For this review, take the finished solid that the model builds, in its own axes (mm). A direction names the side the tool comes from. Coordinates: 2 decimals unless noted, no trailing zeros. Write each loop counter-clockwise with the first axis right and the second up, starting at its lowest first coordinate (ties: lowest second). Pieces come first, ordered by that corner, then holes. Notation, with made-up numbers: (33.25, 55.5) - (39.25, 55.5) arc R33 ccw to (39.25, 88.5) - close; hole circle Ø10 at (52.5, 40). An arc over 180 degrees is marked (long way). Use one line per item in the form item = value. Start each with the question number.
1) We need section C-C (x = 49.5). Give the boundary of the cut face in (y, z).
2) We need section B-B (z = -62). Give the boundary of the cut face in (x, y).
3) Mouldability with a two-part tool opening along X and no side actions: class faces 4 (the cylindrical face through (78.266, 1.521, 80.781)), 5 (the flat face through (1, 0, -1)), 6 (the cylindrical face through (-96.37, 1.48, 72.2)) as pulls with the +X half, pulls with the -X half, needs draft (parallel to the pull), parting line crosses it, or undercut.
4) For L1, parallel to X at y = 0.7, z = -56.5; L2, parallel to X at y = 2.1, z = 62; L3, parallel to X at y = 2.6, z = 23, list the stretches that pass through material, from the lowest coordinate up. Write a range as from..to.
5) We need section A-A (y = 1.35). Give the boundary of the cut face in (x, z).
6) Tool access review of faces 1 (the cylindrical face through (4.322, 1.521, 81.022)), 2 (the cylindrical face through (-4.314, 1.521, -81.101)), 3 (the flat face through (1, 3, -1)): name each direction out of +Z, -Z, +X, -X, +Y, -Y from which nothing blocks a thin tool from reaching the whole face with its end or side.
7) Insertion check: P1, Ø1.5, axis at x = -36.5, y = 2, coming from the -Z side; P2, Ø1.5, axis at y = 2, z = 13, coming from the +X side; P3, Ø1.5, axis at y = 1.5, z = -15, coming from the -X side. Each pin has a flat end and moves straight along its axis. Give the tip position at first contact, or say it passes through.
```python
from build123d import *

# Parameters (mm, degrees)
BOSS_EXTRUDE1_DEPTH = 3
FILLET1_R           = 5.08
FILLET2_R           = 5.08
FILLET3_R           = 5.08


with BuildPart() as part:
    # Sketch1 → Boss-Extrude1 (new body)
    with BuildSketch(Plane(origin=(0, 0, 0), x_dir=(1, 0, 0), z_dir=(0, 1, 0))):
        with BuildLine():
            Line((-76.2, 82.55), (-76.2, 55.95))
            Line((-76.2, 55.95), (-5.842, 55.95))
            Line((-5.842, 55.95), (-5.842, 82.55))
            Line((-5.842, 82.55), (5.770221656, 82.55))
            Line((5.770221656, 82.55), (5.770221656, 55.949868395))
            Line((5.770221656, 55.949868395), (76.2, 55.95))
            Line((76.2, 55.95), (76.2, 82.55))
            ThreePointArc((76.2, 82.55), (94.40904038, 74.510512242), (101.6, 55.95))
            Line((101.6, 55.95), (101.6, -55.95))
            ThreePointArc((101.6, -55.95), (94.40904038, -74.510512242), (76.2, -82.55))
            Line((76.2, -82.55), (76.2, -55.95))
            Line((76.2, -55.95), (5.770221656, -55.95))
            Line((5.770221656, -55.95), (5.770221656, -82.55))
            Line((5.770221656, -82.55), (-5.842, -82.55))
            Line((-5.842, -82.55), (-5.842, -55.95))
            Line((-5.842, -55.95), (-76.2, -55.95))
            Line((-76.2, -55.95), (-76.2, -82.55))
            ThreePointArc((-76.2, -82.55), (-94.40904038, -74.510512242), (-101.6, -55.95))
            Line((-101.6, -55.95), (-101.6, 55.95))
            ThreePointArc((-101.6, 55.95), (-94.40904038, 74.510512242), (-76.2, 82.55))
        make_face()
    extrude(amount=BOSS_EXTRUDE1_DEPTH)

    # Fillet1
    fillet1_edges = [part.edges().sort_by_distance(p)[0] for p in [
        (5.770221656, 1.5, 82.55),
        (-5.842, 1.5, 82.55),
    ]]
    fillet(fillet1_edges, radius=FILLET1_R)

    # Fillet2
    fillet2_edges = [part.edges().sort_by_distance(p)[0] for p in [
        (-5.842, 1.5, -82.55),
        (5.770221656, 1.5, -82.55),
    ]]
    fillet(fillet2_edges, radius=FILLET2_R)

    # Fillet3
    fillet3_edges = [part.edges().sort_by_distance(p)[0] for p in [
        (-76.2, 1.5, -82.55),
        (76.2, 1.5, -82.55),
        (76.2, 1.5, 82.55),
        (-76.2, 1.5, 82.55),
    ]]
    fillet(fillet3_edges, radius=FILLET3_R)


solid = part.part
```
Determined:
q1.outline = (0, -55.95) - (3, -55.95) - (3, 55.95) - (0, 55.95) - close
q2.outline = (-101.03, 0) - (-76.2, 0) - (-76.2, 3) - (-101.03, 3) - close; (-5.84, 0) - (5.77, 0) - (5.77, 3) - (-5.84, 3) - close; (76.2, 0) - (101.03, 0) - (101.03, 3) - (76.2, 3) - close
q3.face_4 = undercut
q3.face_5 = needs draft
q3.face_6 = pulls with the -X half
q4.L1 = -101.61..-76.2, -5.84..5.77, 76.2..101.61
q4.L2 = -101.03..-76.2, -5.84..5.77, 76.2..101.03
q4.L3 = -101.6..101.6
q5.outline = (-101.6, -55.95) arc R26.01 ccw to (-82.66, -81.58) arc R5.08 ccw to (-76.2, -76.69) - (-76.2, -55.95) - (-5.84, -55.95) - (-5.84, -77.47) arc R5.08 ccw to (-0.76, -82.55) - (0.69, -82.55) arc R5.08 ccw to (5.77, -77.47) - (5.77, -55.95) - (76.2, -55.95) - (76.2, -76.69) arc R5.08 ccw to (82.66, -81.58) arc R26.01 ccw to (101.6, -55.95) - (101.6, 55.95) arc R26.01 ccw to (82.66, 81.58) arc R5.08 ccw to (76.2, 76.69) - (76.2, 55.95) - (5.77, 55.95) - (5.77, 77.47) arc R5.08 ccw to (0.69, 82.55) - (-0.76, 82.55) arc R5.08 ccw to (-5.84, 77.47) - (-5.84, 55.95) - (-76.2, 55.95) - (-76.2, 76.69) arc R5.08 ccw to (-82.66, 81.58) arc R26.01 ccw to (-101.6, 55.95) - close
q6.face_1 = +Z, +Y, -Y
q6.face_2 = -Z, +Y, -Y
q6.face_3 = +Z, -Z, +X, -X, +Y
q7.P1 = -55.95
q7.P2 = 101.6
q7.P3 = -101.6
